For this review, take the finished solid that the model builds, in its own axes (mm). Face numbers are marked on the shaded views. A direction names the side the tool comes from. Give positions to 0.01 mm unless a question says otherwise; leave off trailing zeros. Loops run counter-clockwise (first coordinate to the right, second up) from the corner with the lowest first, then second, coordinate; pieces in that order, holes last. Notation, with made-up numbers: (4, 39.25) - (54, 39.25) arc R30 ccw to (54, 66.25) - close; hole circle Ø1 at (46.5, 68.5). An arc over 180 degrees is marked (long way). Answer in a Markdown table with one row per item.
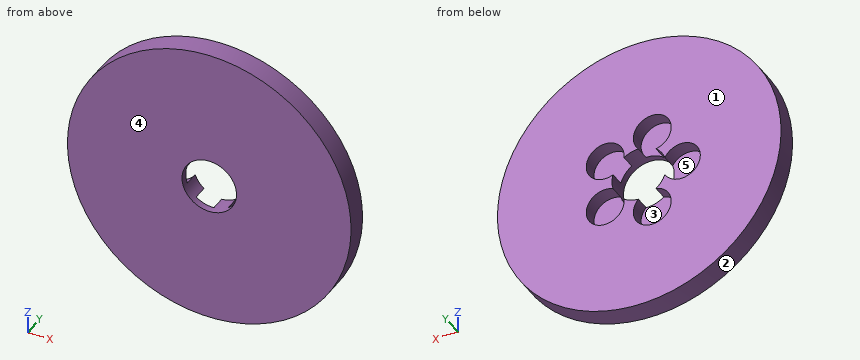
```python
from build123d import *

# Parameters (mm, degrees)
SKETCH1_R           = 65
BOSS_EXTRUDE1_DEPTH = 10
SKETCH2_R           = 12.5
CUT_EXTRUDE1_DEPTH  = 93.466210045
SKETCH3_R           = 8.683348951
CUT_EXTRUDE2_DEPTH  = 6.774962
CIRPATTERN1_START   = 3.225037722
CIRPATTERN1_DEPTH   = 6.774962278


# Read off the part's stored shape, not the designer's step: CirPattern1
with BuildPart() as part:
    # Sketch1 → Boss-Extrude1 (new body)
    with BuildSketch(Plane(origin=(0, 0, 0), x_dir=(1, 0, 0), z_dir=(0, 1, 0))):
        with Locations(Location((0, 0, 0), (0, 0, 270))):
            Circle(SKETCH1_R)
    extrude(amount=BOSS_EXTRUDE1_DEPTH)

    # Sketch2 → Cut-Extrude1 (cut, through all)
    with BuildSketch(Plane(origin=(0, 0, 0), x_dir=(1, 0, 0), z_dir=(0, 1, 0))):
        with Locations(Location((0, 0, 0), (0, 0, 270))):
            Circle(SKETCH2_R)
    extrude(amount=CUT_EXTRUDE1_DEPTH, mode=Mode.SUBTRACT)

    # Sketch3 → Cut-Extrude2 (cut)
    with BuildSketch(Plane(origin=(0, 10, 0), x_dir=(1, 0, 0), z_dir=(0, 1, 0))):
        with Locations((-19.31200649, 0)):
            Circle(SKETCH3_R)
    extrude(amount=-CUT_EXTRUDE2_DEPTH, mode=Mode.SUBTRACT)

    # CirPattern1 outline → CirPattern1 (cut)
    with BuildSketch(Plane(origin=(0, 0, 0), x_dir=(1, 0, 0), z_dir=(0, 1, 0)).offset(CIRPATTERN1_START)):
        with BuildLine():
            ThreePointArc((0.427209526, -12.492697548), (-3.86271243, -11.888206454), (-7.688643147, -9.855697163))
            ThreePointArc((-7.688643147, -9.855697163), (-8.651040595, -26.625165219), (0.427209526, -12.492697548))
        make_face()
        with BuildLine():
            ThreePointArc((0.427209526, 12.492697548), (-8.651040595, 26.625165219), (-7.688643147, 9.855697163))
            ThreePointArc((-7.688643147, 9.855697163), (-3.86271243, 11.888206454), (0.427209526, 12.492697548))
        make_face()
        with BuildLine():
            ThreePointArc((12.013276413, -3.454155444), (10.11271243, -7.347315654), (6.997403613, -10.357912081))
            ThreePointArc((6.997403613, -10.357912081), (22.648718316, -16.455257061), (12.013276413, -3.454155444))
        make_face()
        with BuildLine():
            ThreePointArc((12.013276413, 3.454155444), (22.648718316, 16.455257061), (6.997403613, 10.357912081))
            ThreePointArc((6.997403613, 10.357912081), (10.11271243, 7.347315654), (12.013276413, 3.454155444))
        make_face()
    extrude(amount=CIRPATTERN1_DEPTH, mode=Mode.SUBTRACT)


solid = part.part
```
1. Clearance check with flat-ended pins moving along their axes: pin 1 (2 mm diameter, centred on y = 6, z = 50, fed in from -X); pin 2 (10.5 mm diameter, centred on x = -5.97, z = -18.37, fed in from +Y); pin 3 (3 mm diameter, centred on y = 1.5, z = -38.5, fed in from -X). State where each tip first meets the part, or that it passes through.
Values:
| item | result |
|---|---|
| pin 1 | stops at x = -42.71 |
| pin 2 | stops at y = 3.23 |
| pin 3 | stops at x = -53.44 |
2. We need section B-B, the plane x = -18. Give the boundary of the cut face in (y, z), and give its area (3 significant figures).
Values:
| item | result |
|---|---|
| outline | (0, -62.46) - (10, -62.46) - (10, -8.58) - (3.23, -8.58) - (3.23, 8.58) - (10, 8.58) - (10, 62.46) - (0, 62.46) - close |
| area | 1,130 mm^2 |
3. Mouldability with a two-part tool opening along X and no side actions: class the marked faces 1, 2 and 3 as released by +X, released by -X, zero draft, split by the parting line, or undercut.
Values:
| item | result |
|---|---|
| face 1 | zero draft |
| face 2 | split by the parting line |
| face 3 | undercut |
4. For the marked faces 4 and 5, list the 3-axis set-ups (+Z, -Z, +X, -X, +Y, -Y) from which the entire face can be reached by the end or side of a thin tool; tool diameter is ignored.
Values:
| item | result |
|---|---|
| face 4 | +Z, -Z, +X, -X, -Y |
| face 5 | +Y |
5. We need section C-C, the plane y = 6. Give the boundary of the cut face in (x, z).
Values:
| item | result |
|---|---|
| outline | circle Ø130 at (0, 0); hole (-11.75, -4.27) arc R12.5 ccw to (-7.69, -9.86) arc R8.68 ccw (long way) to (0.43, -12.49) arc R12.5 ccw to (7, -10.36) arc R8.68 ccw (long way) to (12.01, -3.45) arc R12.5 ccw to (12.01, 3.45) arc R8.68 ccw (long way) to (7, 10.36) arc R12.5 ccw to (0.43, 12.49) arc R8.68 ccw (long way) to (-7.69, 9.86) arc R12.5 ccw to (-11.75, 4.27) arc R8.68 ccw (long way) to start |
6. We need section A-A, the plane z = 0. Give the boundary of the cut face in (x, y), and give its area (3 significant figures).
Values:
| item | result |
|---|---|
| outline | (-65, 0) - (-12.5, 0) - (-12.5, 3.23) - (-28, 3.23) - (-28, 10) - (-65, 10) - close; (12.5, 0) - (65, 0) - (65, 10) - (12.5, 10) - close |
| area | 945 mm^2 |
7. We need section D-D, the plane z = -23. Give the boundary of the cut face in (x, y).
Values:
| item | result |
|---|---|
| outline | (-60.79, 0) - (60.79, 0) - (60.79, 10) - (1.38, 10) - (1.38, 3.23) - (-13.31, 3.23) - (-13.31, 10) - (-60.79, 10) - close |
8. Wall thickness on line 1 (X direction, y = 7, z = 16.5); line 2 (X direction, y = 9.75, z = -26); line 3 (X direction, y = 2, z = -11.5): over which ranges is each line inside the solid? List them lowest first. Write a range as [from, to].
Values:
| item | result |
|---|---|
| line 1 | x = [-62.87, -14.45], [2.51, 8.63], [22.62, 62.87] |
| line 2 | x = [-59.57, -10.11], [-1.83, 59.57] |
| line 3 | x = [-63.97, -4.9], [4.9, 63.97] |
